The figure shows three views and two pictorial views of one solid part (mm, origin at its lowest corner). Answer the questions. A direction names the side the tool comes from. Give positions to 0.01 mm unless a question says otherwise; leave off trailing zeros. Loops run counter-clockwise (first coordinate to the right, second up) from the corner with the lowest first, then second, coordinate; pieces in that order, holes last. Notation, with made-up numbers: (-14, -26.5) - (39, -26.5) arc R15 cw to (39, -20.5) - close; hole circle Ø5 at (-2, -15). An arc over 180 degrees is marked (long way). Write each question's results on one line, items separated by ' | '.
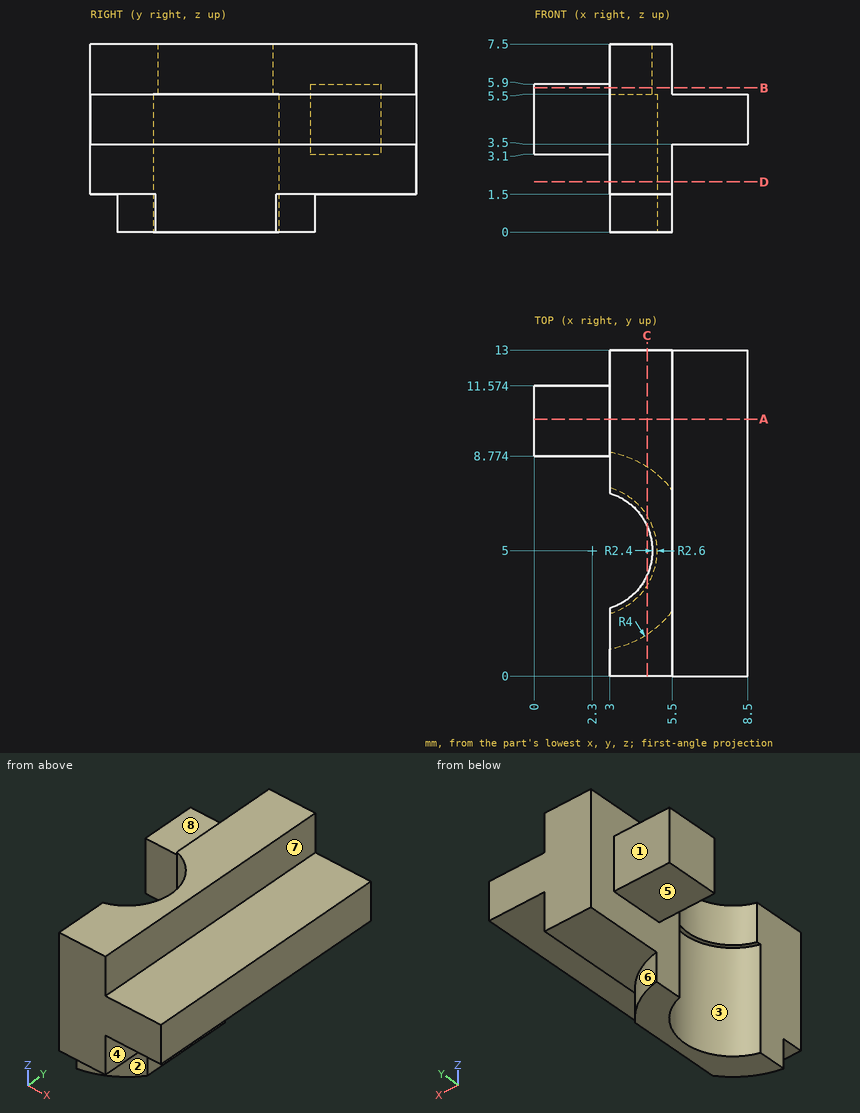
Item 1: A cutting plane is placed at A-A, the plane y = 10.25. Determine the outline of the cut face in (x, z).
Values found:
outline: (0, 3.1) - (3, 3.1) - (3, 1.5) - (5.5, 1.5) - (5.5, 3.5) - (8.5, 3.5) - (8.5, 5.5) - (5.5, 5.5) - (5.5, 7.5) - (3, 7.5) - (3, 5.9) - (0, 5.9) - close
Item 2: For the marked faces 4, 5, 6, 7 and 8, determine the directions among +Z, -Z, +X, -X, +Y, -Y from which every point of the face is accessible in a straight line to the end or side of a thin tool.
Values found:
face 4: -Z, +X, +Y, -Y | face 5: -Z, -X, +Y, -Y | face 6: -Z, +X, +Y | face 7: +Z, +X, +Y, -Y | face 8: +Z, -X, +Y, -Y
Item 3: A cutting plane is placed at C-C, the plane x = 4.5. Determine the outline of the cut face in (y, z) (1 decimal).
Values found:
outline: (0, 1.5) - (1.7, 1.5) - (1.7, 0) - (3.6, 0) - (3.6, 5.5) - (4, 5.5) - (4, 7.5) - (0, 7.5) - close; (6, 5.5) - (6.4, 5.5) - (6.4, 0) - (8.3, 0) - (8.3, 1.5) - (13, 1.5) - (13, 7.5) - (6, 7.5) - close
Item 4: Flat-ended cylindrical pins translate along their axes: P1, Ø2.5, axis at x = 7.5, y = 4.5, coming from the +Z side; P2, Ø3, axis at x = 4, y = 11, coming from the -Z side; P3, Ø0.6, axis at y = 4.5, z = 7, coming from the +X side. Find the tip coordinate at first contact, or state that the pin passes through.
Values found:
P1: stops at z = 5.5 | P2: stops at z = 1.5 | P3: stops at x = 5.5
Item 5: A cutting plane is placed at B-B, the plane z = 5.75. Determine the outline of the cut face in (x, y) (1 decimal).
Values found:
outline: (0, 8.8) - (3, 8.8) - (3, 7.3) arc R2.4 cw to (3, 2.7) - (3, 0) - (5.5, 0) - (5.5, 13) - (3, 13) - (3, 11.6) - (0, 11.6) - close
Item 6: For a pull along Y with two mould halves and no side action, classify the marked faces 1, 2 and 3 as released by +Y, released by -Y, zero draft, split by the parting line, or undercut.
Values found:
face 1: released by +Y | face 2: released by -Y | face 3: undercut
Item 7: A cutting plane is placed at D-D, the plane z = 2. Determine the outline of the cut face in (x, y).
Values found:
outline: (3, 0) - (5.5, 0) - (5.5, 13) - (3, 13) - (3, 7.5) arc R2.6 cw to (3, 2.5) - close
Item 8: Find the intervals of material crossed by line 1 along Z through (x, y) = (7, 3.75); line 2 along X through (y, z) = (11.5, 6.25); line 3 along X through (y, z) = (10.75, 3.25), in increasing order. Write a range as [from, to].
Values found:
line 1: z = [3.5, 5.5] | line 2: x = [3, 5.5] | line 3: x = [0, 5.5]
